from build123d import *

# Parameters (mm, degrees)
F0_R   = 15.875
F0_R_2 = 13.49375


with BuildPart() as f2:
    # F2: sweep along a path in F1
    with BuildLine(Plane.YZ) as f2_path:
        Line((0, 0), (0, 19.05))
        ThreePointArc((0, 19.05), (-2.38381, 28.639399), (-8.980293, 35.996405))
        Line((-8.980293, 35.996405), (-24.743706, 46.693007))
    # F0 (on Top) → F2 (sweep)
    with BuildSketch(Plane.XY):
        with Locations((15.875, 0)):
            Circle(F0_R)
        with Locations((15.875, 0)):
            Circle(F0_R_2, mode=Mode.SUBTRACT)
    sweep(path=f2_path.line)


solid = f2.part
Check sheet for the modelled part. Datum: model origin and axes. Units: mm. Round coordinates to 2 decimals unless told otherwise and drop trailing zeros.
1. Mould release check, pull along Y, two halves, no side actions. Record for faces 1 (the cylindrical face through (31.017, 4.768, 9.658)), 2 (the flat face through (4.19, -20.74, 52.59)), 3 (the cylindrical face through (28.34, -5.17, 9.66)), 4 (the flat face through (9, -12, 0)): released by +Y, released by -Y, zero draft, split by the parting line, or undercut.
2. Scan lines: probe 1 along X at (y, z) = (1.5, 25); probe 2 along X at (y, z) = (6, 18); probe 3 along Y at (x, z) = (10.5, 6). Record each from-to range of solid material in increasing order.
3. Gauge pin test, flat ends, axial feed: pin 1 Ø10 at (x, z) = (13, 22.5) entering from -Y; pin 2 Ø3 at (x, y) = (24.5, 4.5) entering from +Z; pin 3 Ø2 at (x, y) = (11.5, -13.5) entering from +Z; pin 4 Ø6 at (x, y) = (9.5, -16.5) entering from -Z. Record the tip position at first contact, or that the pin passes through.
Recorded:
1. face 1: split by the parting line
1. face 2: released by -Y
1. face 3: undercut
1. face 4: zero draft
2. probe 1: x = 0.17 to 2.58, 29.17 to 31.58
2. probe 2: x = 1.18 to 3.79, 27.96 to 30.57
2. probe 3: y = -14.94 to -12.38, 12.38 to 14.94
3. pin 1: stops at y = -24.39
3. pin 2: stops at z = 43.84
3. pin 3: stops at z = 58.26
3. pin 4: stops at z = 0
